from build123d import *

# Parameters (mm, degrees)
BOSS_EXTRUDE1_DEPTH = 10
SKETCH4_R           = 13.5
CUT_EXTRUDE1_DEPTH  = 4
SKETCH5_R           = 10
CUT_EXTRUDE2_DEPTH  = 78.24797732


with BuildPart() as part:
    # Sketch1 → Boss-Extrude1 (new body)
    with BuildSketch(Plane.XY):
        Polygon((-17.5, 25), (-17.5, 75), (17.5, 75), (17.5, -25), (-17.5, -25), align=None)
    extrude(amount=BOSS_EXTRUDE1_DEPTH)

    # Sketch4 → Cut-Extrude1 (cut)
    with BuildSketch(Plane.XY.offset(10)):
        with Locations((0, 45)):
            Circle(SKETCH4_R)
    extrude(amount=-CUT_EXTRUDE1_DEPTH, mode=Mode.SUBTRACT)

    # Sketch5 → Cut-Extrude2 (cut, through all)
    with BuildSketch(Plane.XY.offset(6)):
        with Locations((0, 45)):
            Circle(SKETCH5_R)
    extrude(amount=-CUT_EXTRUDE2_DEPTH, mode=Mode.SUBTRACT)


solid = part.part
Can you work these out from the model? Positions are in its coordinate system, mm. A direction names the side the tool comes from. Give positions to 0.01 mm unless a question says otherwise; leave off trailing zeros. Loops run counter-clockwise (first coordinate to the right, second up) from the corner with the lowest first, then second, coordinate; pieces in that order, holes last. Notation, with made-up numbers: (62.25, 56) -> (80.25, 56) arc R23 ccw to (80.25, 94) -> close; hole circle Ø7 at (44.25, 80.25). An arc over 180 degrees is marked (long way). Return JSON: item names as keys, results as strings.
Q1. I want a section at D-D, the plane z = 2. List the corners of the cut face in (x, y) for me.
Checks:
{"outline": "(-17.5, -25) -> (17.5, -25) -> (17.5, 75) -> (-17.5, 75) -> close; hole circle Ø20 at (0, 45)"}
Q2. We'd pull the mould along Y, two halves only. Please class faces 1 (the face through (-2.17, 35.24, 3.04)), 2 (the face through (0, 75, 5)), 3 (the face through (17.5, 26, 5)), 4 (the face through (-1.757, 58.385, 8.028)): released by +Y, released by -Y, zero draft, split by the parting line, or undercut.
Checks:
{"face 1": "undercut", "face 2": "released by +Y", "face 3": "zero draft", "face 4": "undercut"}
Q3. I want a section at B-B, the plane y = 45. List the corners of the cut face in (x, z) for me, then the cut area to 3 significant figures.
Checks:
{"outline": "(-17.5, 0) -> (-10, 0) -> (-10, 6) -> (-13.5, 6) -> (-13.5, 10) -> (-17.5, 10) -> close; (10, 0) -> (17.5, 0) -> (17.5, 10) -> (13.5, 10) -> (13.5, 6) -> (10, 6) -> close", "area": "122 mm2"}
Q4. For pin 1 Ø8 at (x, y) = (2.5, 39.5) entering from +Z, with a flat end and sliding along its axis, tell me the tip position at first contact or that it passes through.
Checks:
{"pin 1": "stops at z = 6"}
Q5. I want a section at A-A, the plane x = 0. List the corners of the cut face in (y, z) for me.
Checks:
{"outline": "(-25, 0) -> (35, 0) -> (35, 6) -> (31.5, 6) -> (31.5, 10) -> (-25, 10) -> close; (55, 0) -> (75, 0) -> (75, 10) -> (58.5, 10) -> (58.5, 6) -> (55, 6) -> close"}
Q6. I want a section at C-C, the plane z = 7.75. List the corners of the cut face in (x, y) for me.
Checks:
{"outline": "(-17.5, -25) -> (17.5, -25) -> (17.5, 75) -> (-17.5, 75) -> close; hole circle Ø27 at (0, 45)"}
Q7. On a 3-axis mill with a long thin cutter (end or side, diameter ignored), from which of +Z, -Z, +X, -X, +Y, -Y can I reach the whole of each face in a straight line? I mean faces 5 (the face through (-9, 40, 6)), 6 (the face through (-17.5, 26, 5)). Say none if no direction works.
Checks:
{"face 5": "+Z", "face 6": "+Z, -Z, -X, +Y, -Y"}
Q8. I need wall thicknesses on probe 1 along Y at (x, z) = (0, 8.7); probe 2 along Y at (x, z) = (0, 3.7); probe 3 along X at (y, z) = (53, 8.75). Which ranges of each line are inside material? Lowest first, please.
Checks:
{"probe 1": "y = -25 to 31.5, 58.5 to 75", "probe 2": "y = -25 to 35, 55 to 75", "probe 3": "x = -17.5 to -10.87, 10.87 to 17.5"}
